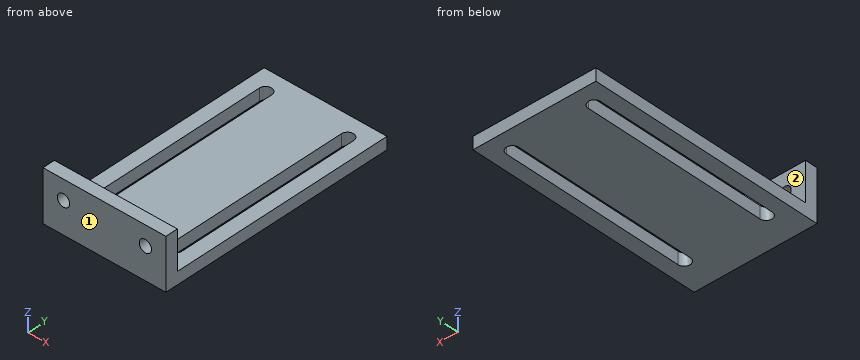
from build123d import *

# Parameters (mm, degrees)
SKETCH1_W           = 30
SKETCH1_H           = 12.5
BOSS_EXTRUDE1_DEPTH = 3
SKETCH2_W           = 30
SKETCH2_H           = 3
BOSS_EXTRUDE2_DEPTH = 55
CUT_EXTRUDE1_DEPTH  = 4
SKETCH4_R           = 1.5
CUT_EXTRUDE2_DEPTH  = 4


with BuildPart() as part:
    # Sketch1 → Boss-Extrude1 (new body)
    with BuildSketch(Plane(origin=(0, 0, 0), x_dir=(1, 0, 0), z_dir=(0, 1, 0))):
        Rectangle(SKETCH1_W, SKETCH1_H)
    extrude(amount=BOSS_EXTRUDE1_DEPTH)

    # Sketch2 → Boss-Extrude2 (add)
    with BuildSketch(Plane(origin=(0, 3, 0), x_dir=(1, 0, 0), z_dir=(0, 1, 0))):
        with Locations((0, 4.75)):
            Rectangle(SKETCH2_W, SKETCH2_H)
    extrude(amount=BOSS_EXTRUDE2_DEPTH)

    # Sketch3 → Cut-Extrude1 (cut, through all)
    with BuildSketch(Plane.XY.offset(-3.25)):
        with BuildLine():
            Line((-8.5, 53), (-8.5, 8))
            ThreePointArc((-8.5, 8), (-10, 6.5), (-11.5, 8))
            Line((-11.5, 8), (-11.5, 53))
            ThreePointArc((-11.5, 53), (-10, 54.5), (-8.5, 53))
        make_face()
        with BuildLine():
            Line((8.5, 53), (8.5, 8))
            ThreePointArc((8.5, 8), (10, 6.5), (11.5, 8))
            Line((11.5, 8), (11.5, 53))
            ThreePointArc((11.5, 53), (10, 54.5), (8.5, 53))
        make_face()
    extrude(amount=-CUT_EXTRUDE1_DEPTH, mode=Mode.SUBTRACT)

    # Sketch4 → Cut-Extrude2 (cut, through all)
    with BuildSketch(Plane(origin=(0, 3, 0), x_dir=(1, 0, 0), z_dir=(0, 1, 0))):
        with Locations((-10, -1.5)):
            Circle(SKETCH4_R)
        with Locations((10, -1.5)):
            Circle(SKETCH4_R)
    extrude(amount=-CUT_EXTRUDE2_DEPTH, mode=Mode.SUBTRACT)


solid = part.part
The listing builds one solid part. Answer for the finished solid, in the listing's coordinates (mm). Face numbers are marked on the shaded views. A direction names the side the tool comes from. Round coordinates to 2 decimals unless told otherwise and drop trailing zeros. Write each loop counter-clockwise with the first axis right and the second up, starting at its lowest first coordinate (ties: lowest second). Pieces come first, ordered by that corner, then holes. Notation, with made-up numbers: M 4.5,20.25 L 17.5,20.25 A20 cw 17.5,42.25 Z; hole C -18.75,-23 d11. An arc over 180 degrees is marked long. Write each question's results on one line, items separated by ' | '. Start each with the question number.
Item 1: A cutting plane is placed at A-A on z = 1.5. Write down the section's boundary in (x, y), and give its area (3 significant figures).
Item 2: Straight lines are drawn through the part: L1, parallel to X at y = 1.8, z = 1.5; L2, parallel to Y at x = -10, z = -5.5; L3, parallel to Z at x = 10, y = 1.9. For each, find the intervals that lie inside material, in ascending order. Write a range as [from, to].
Item 3: A cutting plane is placed at D-D on z = -4.5. Write down the section's boundary in (x, y).
Item 4: A cutting plane is placed at B-B on y = 29. Write down the section's boundary in (x, z).
Item 5: A cutting plane is placed at C-C on x = 10. Write down the section's boundary in (y, z), and give its area (3 significant figures).
Item 6: Flat-ended cylindrical pins translate along their axes: pin 1 Ø4 at (x, z) = (8.5, 0) entering from +Y; pin 2 Ø1 at (x, z) = (10.5, 1) entering from +Y; pin 3 Ø10 at (x, y) = (8.5, 13.5) entering from +Z. Find the tip coordinate at first contact, or state that the pin passes through.
Item 7: For the marked faces 1 and 2, determine the directions among +Z, -Z, +X, -X, +Y, -Y from which every point of the face is accessible in a straight line to the end or side of a thin tool.
Check sheet entries:
1) outline: M -15,0 L -11.5,0 L -11.5,3 L -15,3 Z; M -8.5,0 L 8.5,0 L 8.5,3 L -8.5,3 Z; M 11.5,0 L 15,0 L 15,3 L 11.5,3 Z | area: 72.0 mm²
2) L1: [-15, -11.5], [-8.5, 8.5], [11.5, 15] | L2: [0, 6.5], [54.5, 58] | L3: [-6.25, 0], [3, 6.25]
3) outline: M -15,0 L 15,0 L 15,58 L -15,58 Z; hole M -11.5,8 A1.5 ccw -8.5,8 L -8.5,53 A1.5 ccw -11.5,53 Z; hole M 8.5,8 A1.5 ccw 11.5,8 L 11.5,53 A1.5 ccw 8.5,53 Z
4) outline: M -15,-6.25 L -11.5,-6.25 L -11.5,-3.25 L -15,-3.25 Z; M -8.5,-6.25 L 8.5,-6.25 L 8.5,-3.25 L -8.5,-3.25 Z; M 11.5,-6.25 L 15,-6.25 L 15,-3.25 L 11.5,-3.25 Z
5) outline: M 0,-6.25 L 6.5,-6.25 L 6.5,-3.25 L 3,-3.25 L 3,0 L 0,0 Z; M 0,3 L 3,3 L 3,6.25 L 0,6.25 Z; M 54.5,-6.25 L 58,-6.25 L 58,-3.25 L 54.5,-3.25 Z | area: 49.5 mm²
6) pin 1: y = 3 | pin 2: through | pin 3: z = -3.25
7) face 1: +Z, -Z, +X, -X, -Y | face 2: +Z, +X, -X, +Y
